from build123d import *


with BuildPart() as part:
    # Esquisse1 → Base-Révolution (revolve)
    with BuildSketch(Plane.XY, mode=Mode.PRIVATE) as base_r_volution_sk:
        with BuildLine():
            Line((5, 0), (5, 9.2))
            ThreePointArc((5, 9.2), (5.527207794, 10.472792206), (6.8, 11))
            Line((6.8, 11), (9, 11))
            Line((9, 11), (9, 9))
            Line((9, 9), (7.8, 9))
            ThreePointArc((7.8, 9), (7.234314575, 8.765685425), (7, 8.2))
            Line((7, 8.2), (7, 0))
            Line((7, 0), (5, 0))
        make_face()
    revolve(base_r_volution_sk.sketch.rotate(Axis((0, 0, 0), (0, 1, 0)), 90), axis=Axis((0, 0, 0), (0, 1, 0)))


solid = part.part
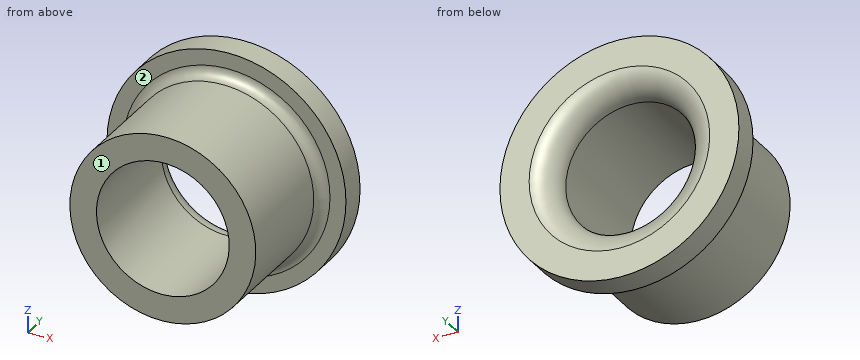
Could you check a few things on this model? Use its own coordinates, in mm. Face numbers are marked on the shaded views. A direction names the side the tool comes from. Give positions to 0.01 mm unless a question says otherwise; leave off trailing zeros. Loops run counter-clockwise (first coordinate to the right, second up) from the corner with the lowest first, then second, coordinate; pieces in that order, holes last. Notation, with made-up numbers: (12, 10) -> (59, 10) arc R25 ccw to (59, 43) -> close; hole circle Ø11 at (-1, 26.5). An arc over 180 degrees is marked (long way). Return JSON: item names as keys, results as strings.
Item 1: If we section it at A-A on x = 0: List the corners of the cut face in (y, z) for me, plus the area to 3 significant figures.
Geometry results:
{"outline": "(0, -7) -> (8.2, -7) arc R0.8 cw to (9, -7.8) -> (9, -9) -> (11, -9) -> (11, -6.8) arc R1.8 ccw to (9.2, -5) -> (0, -5) -> close; (0, 5) -> (9.2, 5) arc R1.8 ccw to (11, 6.8) -> (11, 9) -> (9, 9) -> (9, 7.8) arc R0.8 cw to (8.2, 7) -> (0, 7) -> close", "area": "50.9 mm²"}
Item 2: If we section it at C-C on y = 8.5: List the corners of the cut face in (x, z) for me.
Geometry results:
{"outline": "circle Ø14.12 at (0, 0); hole circle Ø10 at (0, 0)"}
Item 3: I need wall thicknesses on L1, parallel to X at y = 2.5, z = 0; L2, parallel to Y at x = -7.5, z = -4.25; L3, parallel to Z at x = -1.25, y = 5.75. Which ranges of each line are inside material? Lowest first, please. Write a range as from..to.
Geometry results:
{"L1": "x = -7..-5, 5..7", "L2": "y = 9..11", "L3": "z = -6.89..-4.84, 4.84..6.89"}
Item 4: If we section it at B-B on z = 0: List the corners of the cut face in (x, y) for me.
Geometry results:
{"outline": "(-9, 9) -> (-7.8, 9) arc R0.8 cw to (-7, 8.2) -> (-7, 0) -> (-5, 0) -> (-5, 9.2) arc R1.8 ccw to (-6.8, 11) -> (-9, 11) -> close; (5, 0) -> (7, 0) -> (7, 8.2) arc R0.8 cw to (7.8, 9) -> (9, 9) -> (9, 11) -> (6.8, 11) arc R1.8 ccw to (5, 9.2) -> close"}
Item 5: Which directions (+Z, -Z, +X, -X, +Y, -Y) give clear straight access to the entire face, cutting with the end or side of a thin tool? Please do the marked faces 1 and 2.
Geometry results:
{"face 1": "+Z, -Z, +X, -X, -Y", "face 2": "-Y"}
Item 6: I'm going to push flat-ended pins straight in: pin 1 (4 mm diameter, centred on y = 9, z = -6.5, fed in from +X); pin 2 (6 mm diameter, centred on x = 4, y = 2.5, fed in from +Z); pin 3 (5 mm diameter, centred on x = -2, y = 3.5, fed in from +Z); pin 4 (8 mm diameter, centred on x = 0, z = 0, fed in from +Y). Where does each tip first touch, or does it pass through?
Geometry results:
{"pin 1": "stops at x = 7.79", "pin 2": "stops at z = 6.93", "pin 3": "stops at z = 7", "pin 4": "passes through"}
